from build123d import *

# Parameters (mm, degrees)
ESQUISSE1_W             = 165
ESQUISSE1_H             = 120
BOSS_EXTRU_1_DEPTH      = 4
ESQUISSE2_R             = 2
ESQUISSE2_R_2           = 1.5
ESQUISSE2_W             = 20
ESQUISSE2_H             = 30
ENL_V_MAT_EXTRU_1_DEPTH = 176.616058491
CONG_1_R                = 3
CONG_2_R                = 6.5
ESQUISSE3_R             = 1
ENL_V_MAT_EXTRU_2_DEPTH = 176.616058491
ESQUISSE4_R             = 2.5
ESQUISSE4_R_2           = 1
ENL_V_MAT_EXTRU_3_DEPTH = 176.616058491
ESQUISSE6_R             = 0.5
ESQUISSE6_W             = 50
ESQUISSE6_H             = 40
ENL_V_MAT_EXTRU_4_DEPTH = 176.616058491
CONG_3_R                = 5


with BuildPart() as part:
    # Esquisse1 → Boss.-Extru.1 (new body)
    with BuildSketch(Plane(origin=(0, 0, 0), x_dir=(1, 0, 0), z_dir=(0, 1, 0))):
        with Locations((82.5, 0)):
            Rectangle(ESQUISSE1_W, ESQUISSE1_H)
    extrude(amount=BOSS_EXTRU_1_DEPTH)

    # Esquisse2 → Enlèv. mat.-Extru.1 (cut, through all)
    with BuildSketch(Plane(origin=(0, 4, 0), x_dir=(1, 0, 0), z_dir=(0, 1, 0))):
        with Locations(Location((55, 25, 0), (0, 0, 270))):
            Circle(ESQUISSE2_R)
        with Locations(Location((88, 25, 0), (0, 0, 270))):
            Circle(ESQUISSE2_R)
        with Locations(Location((88, -25, 0), (0, 0, 90))):
            Circle(ESQUISSE2_R)
        with Locations(Location((55, -25, 0), (0, 0, 90))):
            Circle(ESQUISSE2_R)
        with Locations(Location((55, -37.5, 0), (0, 0, 270))):
            Circle(ESQUISSE2_R_2)
        with Locations(Location((88, -37.5, 0), (0, 0, 270))):
            Circle(ESQUISSE2_R_2)
        with Locations(Location((123, -37.5, 0), (0, 0, 270))):
            Circle(ESQUISSE2_R_2)
        with Locations(Location((123, 37.5, 0), (0, 0, 90))):
            Circle(ESQUISSE2_R_2)
        with Locations(Location((88, 37.5, 0), (0, 0, 90))):
            Circle(ESQUISSE2_R_2)
        with Locations(Location((55, 37.5, 0), (0, 0, 90))):
            Circle(ESQUISSE2_R_2)
        Polygon((126, -25), (126, -32.5), (92, -32.5), (92, 32.5), (126, 32.5), (126, 25), (159, 25), (159, -25), align=None)
        with Locations((71.5, 0)):
            Rectangle(ESQUISSE2_W, ESQUISSE2_H)
    extrude(amount=-ENL_V_MAT_EXTRU_1_DEPTH, mode=Mode.SUBTRACT)

    # Congé1
    cong_1_edges = [part.edges().sort_by_distance(p)[0] for p in [
        (92, 2, 32.5),
        (92, 2, -32.5),
        (126, 2, -32.5),
        (126, 2, -25),
        (159, 2, -25),
        (159, 2, 25),
        (126, 2, 25),
        (126, 2, 32.5),
        (61.5, 2, 15),
        (61.5, 2, -15),
        (81.5, 2, -15),
        (81.5, 2, 15),
    ]]
    fillet(cong_1_edges, radius=CONG_1_R)

    # Congé2
    cong_2_edges = [part.edges().sort_by_distance(p)[0] for p in [
        (165, 2, -60),
        (165, 2, 60),
    ]]
    fillet(cong_2_edges, radius=CONG_2_R)

    # Esquisse3 → Enlèv. mat.-Extru.2 (cut, through all)
    with BuildSketch(Plane(origin=(0, 4, 0), x_dir=(1, 0, 0), z_dir=(0, 1, 0))):
        with Locations(Location((158.5, -53.5, 0), (0, 0, 270))):
            Circle(ESQUISSE3_R)
        with Locations(Location((158.5, 53.5, 0), (0, 0, 270))):
            Circle(ESQUISSE3_R)
        with Locations(Location((156, 32.5, 0), (0, 0, 270))):
            Circle(ESQUISSE3_R)
        with Locations(Location((156, -32.5, 0), (0, 0, 90))):
            Circle(ESQUISSE3_R)
    extrude(amount=-ENL_V_MAT_EXTRU_2_DEPTH, mode=Mode.SUBTRACT)

    # Esquisse4 → Enlèv. mat.-Extru.3 (cut, through all)
    with BuildSketch(Plane(origin=(0, 4, 0), x_dir=(1, 0, 0), z_dir=(0, 1, 0))):
        with Locations(Location((120, -50, 0), (0, 0, 270))):
            Circle(ESQUISSE4_R)
        with Locations(Location((38, -50, 0), (0, 0, 270))):
            Circle(ESQUISSE4_R)
        with Locations(Location((38, 50, 0), (0, 0, 90))):
            Circle(ESQUISSE4_R)
        with Locations(Location((120, 50, 0), (0, 0, 90))):
            Circle(ESQUISSE4_R)
        with Locations((0, 45)):
            Circle(ESQUISSE4_R_2)
        with Locations(Location((70, 45, 0), (0, 0, 270))):
            Circle(ESQUISSE4_R_2)
        with Locations(Location((140, 45, 0), (0, 0, 270))):
            Circle(ESQUISSE4_R_2)
        with Locations(Location((140, -45, 0), (0, 0, 90))):
            Circle(ESQUISSE4_R_2)
        with Locations(Location((70, -45, 0), (0, 0, 90))):
            Circle(ESQUISSE4_R_2)
        with Locations((0, -45)):
            Circle(ESQUISSE4_R_2)
    extrude(amount=-ENL_V_MAT_EXTRU_3_DEPTH, mode=Mode.SUBTRACT)

    # Symétrie1: part across plane


with BuildPart() as part_1:
    add(part.part)
    add(part.part.mirror(Plane(origin=(0, 4, -60), x_dir=(0, 0, 1), z_dir=(1, 0, 0))))

    # Esquisse6 → Enlèv. mat.-Extru.4 (cut, through all)
    with BuildSketch(Plane(origin=(0, 4, 0), x_dir=(1, 0, 0), z_dir=(0, 1, 0))):
        with Locations((165, 0)):
            Circle(ESQUISSE6_R)
        with Locations((-165, 0)):
            Circle(ESQUISSE6_R)
        Rectangle(ESQUISSE6_W, ESQUISSE6_H)
    extrude(amount=-ENL_V_MAT_EXTRU_4_DEPTH, mode=Mode.SUBTRACT)

    # Congé3
    cong_3_edges = [part_1.edges().sort_by_distance(p)[0] for p in [
        (25, 2, -20),
        (25, 2, 20),
        (-25, 2, 20),
        (-25, 2, -20),
    ]]
    fillet(cong_3_edges, radius=CONG_3_R)


solid = part_1.part
Source: CAD feature listing. Evaluate the final solid. Frame: model axes, mm. Coordinates: 2 decimals unless noted, no trailing zeros. Loops run counter-clockwise (first coordinate to the right, second up) from the corner with the lowest first, then second, coordinate; pieces in that order, holes last. Notation, with made-up numbers: (17, 50) - (72, 50) arc R22 cw to (72, 75) - close; hole circle Ø7 at (46.25, -36.5). An arc over 180 degrees is marked (long way). Return JSON: item names as keys, results as strings.
Q1. Section B-B, the plane y = 0.6. Give the number of separate pieces and of enclosed holes in the cut face, plus the area to 3 significant figures.
Results:
{"separate pieces": "1", "enclosed holes": "51", "area": "28,300 mm2"}
Q2. Material intervals for line 1 along X through (y, z) = (1.35, -2); line 2 along X through (y, z) = (0.85, -19); line 3 along X through (y, z) = (1.8, -29.5), sorted ascending.
Results:
{"line 1": "-165 to -159, -92 to -81.5, -61.5 to -25, 25 to 61.5, 81.5 to 92, 159 to 165", "line 2": "-165 to -159, -92 to -23, 23 to 92, 159 to 165", "line 3": "-165 to -126, -92 to 92, 126 to 165"}
Q3. Section A-A, the plane z = 7. Return loops of the section in (x, y), plus the area to 3 significant figures.
Results:
{"outline": "(-165, 0) - (-159, 0) - (-159, 4) - (-165, 4) - close; (-92, 0) - (-81.5, 0) - (-81.5, 4) - (-92, 4) - close; (-61.5, 0) - (-25, 0) - (-25, 4) - (-61.5, 4) - close; (25, 0) - (61.5, 0) - (61.5, 4) - (25, 4) - close; (81.5, 0) - (92, 0) - (92, 4) - (81.5, 4) - close; (159, 0) - (165, 0) - (165, 4) - (159, 4) - close", "area": "424 mm2"}
Q4. Mould query, pull axis X, two halves, no side actions, for faces 1 (the flat face through (2, 0, -28)), 2 (the cylindrical face through (163.045, 2.028, 58.146)), 3 (the cylindrical face through (-163.045, 2.028, 58.146)). Classes: released by +X, released by -X, zero draft, split by the parting line, or undercut.
Results:
{"face 1": "zero draft", "face 2": "released by +X", "face 3": "released by -X"}
